Part model, mm, in its own coordinate system. Coordinates: 2 decimals unless noted, no trailing zeros. Order: outer loops, then holes, each group sorted by start corner. A loop starts at its lowest first (then second) coordinate and runs counter-clockwise, first axis right, second up.
1) Wall check: L1, parallel to X at y = -13.5, z = 23.5; L2, parallel to Y at x = 10, z = 23 (3 decimals); L3, parallel to Z at x = 8, y = 3. Give the ranges that are in metal, low to high.
2) Cut at A-A (x = 1.5). List the corners of the cut face in (y, z) (3 decimals).
3) Pin check, flat tip, straight feed: pin 1 Ø4 at (x, y) = (-11, -13) entering from -Z. Stop position of the tip, or through.
```python
from build123d import *

# Parameters (mm, degrees)
F0_W     = 38.1
F0_H     = 38.1
F1_DEPTH = 25.4
F3_DEPTH = 2.54


with BuildPart() as f1:
    # F0 (on Top) → F1 (new body)
    with BuildSketch(Plane.XY):
        Rectangle(F0_W, F0_H)
    extrude(amount=F1_DEPTH)

    # F2 (on face) → F3 (cut)
    with BuildSketch(Plane.XY.offset(25.4)):
        with BuildLine():
            Line((-13.97, -6.985), (-13.97, -13.97))
            ThreePointArc((-13.97, -13.97), (-13.335, -14.605), (-12.7, -13.97))
            Line((-12.7, -13.97), (-12.7, -8.255))
            Line((-12.7, -8.255), (8.89, -8.255))
            Line((8.89, -8.255), (8.89, -3.175))
            Line((8.89, -3.175), (-7.62, -3.175))
            Line((-7.62, -3.175), (-7.62, -0.635))
            Line((-7.62, -0.635), (8.89, -0.635))
            Line((8.89, -0.635), (8.89, 4.445))
            Line((8.89, 4.445), (-7.62, 4.445))
            Line((-7.62, 4.445), (-7.62, 6.985))
            Line((-7.62, 6.985), (13.97, 6.985))
            Line((13.97, 6.985), (13.97, 13.97))
            ThreePointArc((13.97, 13.97), (13.335, 14.605), (12.7, 13.97))
            Line((12.7, 13.97), (12.7, 8.255))
            Line((12.7, 8.255), (-8.89, 8.255))
            Line((-8.89, 8.255), (-8.89, 3.175))
            Line((-8.89, 3.175), (7.62, 3.175))
            Line((7.62, 3.175), (7.62, 0.635))
            Line((7.62, 0.635), (-8.89, 0.635))
            Line((-8.89, 0.635), (-8.89, -4.445))
            Line((-8.89, -4.445), (7.62, -4.445))
            Line((7.62, -4.445), (7.62, -6.985))
            Line((7.62, -6.985), (-13.97, -6.985))
        make_face()
    extrude(amount=-F3_DEPTH, mode=Mode.SUBTRACT)


solid = f1.part
```
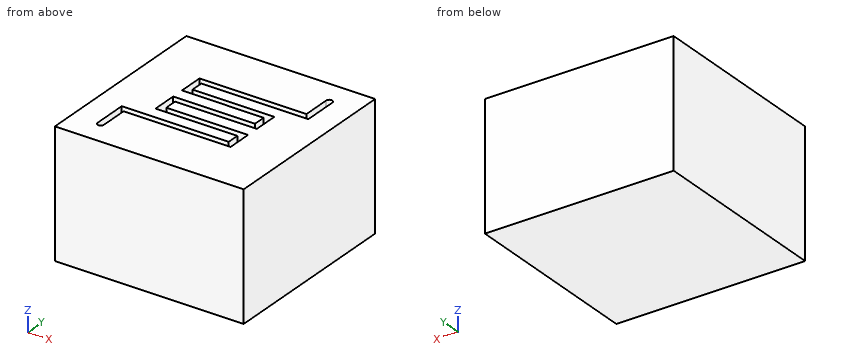
Geometry check:
1. L1: x = -19.05 to -13.97, -12.7 to 19.05
1. L2: y = -19.05 to 6.985, 8.255 to 19.05
1. L3: z = 0 to 22.86
2. outline: (-19.05, 0) - (19.05, 0) - (19.05, 25.4) - (8.255, 25.4) - (8.255, 22.86) - (6.985, 22.86) - (6.985, 25.4) - (4.445, 25.4) - (4.445, 22.86) - (3.175, 22.86) - (3.175, 25.4) - (0.635, 25.4) - (0.635, 22.86) - (-0.635, 22.86) - (-0.635, 25.4) - (-3.175, 25.4) - (-3.175, 22.86) - (-4.445, 22.86) - (-4.445, 25.4) - (-6.985, 25.4) - (-6.985, 22.86) - (-8.255, 22.86) - (-8.255, 25.4) - (-19.05, 25.4) - close
3. pin 1: stops at z = 0
